Geometry check sheet. Reference: the model listing, model coordinates, mm. Face numbers are marked on the shaded views. A direction names the side the tool comes from. Round coordinates to 2 decimals unless told otherwise and drop trailing zeros. Write each loop counter-clockwise with the first axis right and the second up, starting at its lowest first coordinate (ties: lowest second). Pieces come first, ordered by that corner, then holes. Notation, with made-up numbers: (47.5, 0.25) - (53.5, 0.25) arc R28 ccw to (53.5, 33.25) - close; hole circle Ø9 at (88, 43.25). An arc over 180 degrees is marked (long way). Return JSON: item names as keys, results as strings. Group by question number.
from build123d import *

# Parameters (mm, degrees)
CROQUIS1_R                 = 13
SALIENTE_EXTRUIR1_DEPTH    = 62
CROQUIS2_R                 = 5
CORTAR_EXTRUIR1_DEPTH      = 62
CROQUIS3_R                 = 2.5
CORTAR_EXTRUIR2_DEPTH      = 62
CORTAR_EXTRUIR2_DEPTH_BACK = 62
SALIENTE_EXTRUIR2_DEPTH    = 62
CROQUIS5_W                 = 52
CROQUIS5_H                 = 35
CORTAR_EXTRUIR4_DEPTH      = 62
CROQUIS6_R                 = 2.5
CORTAR_EXTRUIR5_DEPTH      = 62
CROQUIS7_R                 = 5
CORTAR_EXTRUIR6_DEPTH      = 62
CORTAR_EXTRUIR8_DEPTH      = 62
CORTAR_EXTRUIR8_DEPTH_BACK = 62


with BuildPart() as part:
    # Croquis1 → Saliente-Extruir1 (new body)
    with BuildSketch(Plane(origin=(0, 0, 0), x_dir=(0, 0, -1), z_dir=(1, 0, 0))):
        Circle(CROQUIS1_R)
    extrude(amount=SALIENTE_EXTRUIR1_DEPTH)

    # Croquis2 → Cortar-Extruir1 (cut)
    with BuildSketch(Plane(origin=(62, 0, 0), x_dir=(0, 0, -1), z_dir=(1, 0, 0))):
        Circle(CROQUIS2_R)
    extrude(amount=-CORTAR_EXTRUIR1_DEPTH, mode=Mode.SUBTRACT)

    # Croquis3 → Cortar-Extruir2 (cut, two sides)
    with BuildSketch(Plane(origin=(0, 0, 0), x_dir=(1, 0, 0), z_dir=(0, 1, 0))) as cortar_extruir2_sk:
        with Locations((31, 0)):
            Circle(CROQUIS3_R)
    extrude(amount=CORTAR_EXTRUIR2_DEPTH, mode=Mode.SUBTRACT)
    extrude(cortar_extruir2_sk.sketch, amount=-CORTAR_EXTRUIR2_DEPTH_BACK, mode=Mode.SUBTRACT)

    # Croquis4 → Saliente-Extruir2 (add)
    with BuildSketch(Plane(origin=(62, 0, 0), x_dir=(0, 0, -1), z_dir=(1, 0, 0))):
        with BuildLine():
            Line((50, 13), (0, 13))
            ThreePointArc((0, 13), (13, 0), (0, -13))
            Line((0, -13), (50, -13))
            Line((50, -13), (80, -5))
            Line((80, -5), (80, 0))
            Line((80, 0), (80, 5))
            Line((80, 5), (50, 13))
        make_face()
    extrude(amount=-SALIENTE_EXTRUIR2_DEPTH)

    # Croquis5 → Cortar-Extruir4 (cut)
    with BuildSketch(Plane(origin=(0, 13, 0), x_dir=(1, 0, 0), z_dir=(0, 1, 0))):
        with Locations((31, 27.5)):
            Rectangle(CROQUIS5_W, CROQUIS5_H)
    extrude(amount=-CORTAR_EXTRUIR4_DEPTH, mode=Mode.SUBTRACT)

    # Croquis6 → Cortar-Extruir5 (cut)
    with BuildSketch(Plane(origin=(0, 13, 0), x_dir=(1, 0, 0), z_dir=(0, 1, 0))):
        with Locations((31, 0)):
            Circle(CROQUIS6_R)
    extrude(amount=-CORTAR_EXTRUIR5_DEPTH, mode=Mode.SUBTRACT)

    # Croquis7 → Cortar-Extruir6 (cut)
    with BuildSketch(Plane(origin=(0, 0, -80), x_dir=(-1, 0, 0), z_dir=(0, 0, -1))):
        with Locations((-31, 0)):
            Circle(CROQUIS7_R)
    extrude(amount=-CORTAR_EXTRUIR6_DEPTH, mode=Mode.SUBTRACT)

    # Croquis8 → Cortar-Extruir8 (cut, two sides)
    with BuildSketch(Plane(origin=(0, 0, 0), x_dir=(1, 0, 0), z_dir=(0, 1, 0))) as cortar_extruir8_sk:
        Polygon((0, 50), (0, 80), (21, 80), align=None)
        Polygon((41, 80), (62, 50), (62, 80), align=None)
        Polygon((41, 80), (41, 50), (62, 50), align=None)
        Polygon((21, 80), (21, 50), (0, 50), align=None)
    extrude(amount=CORTAR_EXTRUIR8_DEPTH, mode=Mode.SUBTRACT)
    extrude(cortar_extruir8_sk.sketch, amount=-CORTAR_EXTRUIR8_DEPTH_BACK, mode=Mode.SUBTRACT)


solid = part.part
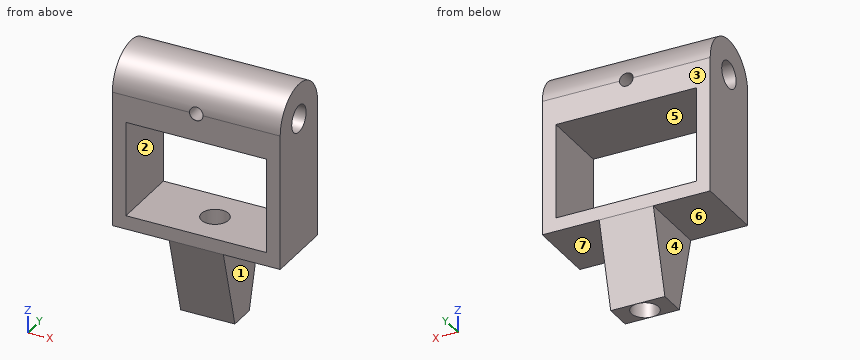
1. Material ranges on line 1 along X through (y, z) = (6.5, 0); line 2 along X through (y, z) = (0, -55.5); line 3 along Y through (x, z) = (47, 0), recorded low to high.
2. Section check B-B (z = -42.5). Enter the section's corners in (x, y).
3. Section check C-C (y = 0). Enter the section's corners in (x, z), and give its area (3 significant figures).
4. Section check A-A (x = 51.5). Enter the section's corners in (y, z), and give its area (3 significant figures).
5. Mould release check, pull along X, two halves, no side actions. Record for the marked faces 1, 2, 3 and 4: pulls with the +X half, pulls with the -X half, needs draft (parallel to the pull), parting line crosses it, or undercut.
6. Tool access check on the marked faces 5, 6 and 7. Record the directions out of +Z, -Z, +X, -X, +Y, -Y that give a thin tool (end or side, any length) a straight path to the whole face; none if there is none.
7. Section check D-D (z = -4). Enter the section's corners in (x, y).
8. Depth check by flat-ended pin: pin 1 Ø3 at (x, z) = (31, 0) entering from +Y; pin 2 Ø3 at (x, z) = (38, 1) entering from -Y; pin 3 Ø13 at (y, z) = (1, -65.5) entering from -X; pin 4 Ø6 at (y, z) = (0, -69) entering from +X. Enter the tip coordinate at first touch or a pass-through.
Result sheet:
{
 "1": {"line 1": "x = 0 to 28.5, 33.5 to 62", "line 2": "x = 21 to 26, 36 to 41", "line 3": "y = -13 to -5, 5 to 13"},
 "2": {"outline": "(0, -13) - (5, -13) - (5, 13) - (0, 13) - close; (57, -13) - (62, -13) - (62, 13) - (57, 13) - close"},
 "3": {"outline": "(0, -50) - (21, -50) - (21, -80) - (26, -80) - (26, -45) - (5, -45) - (5, -10) - (57, -10) - (57, -45) - (36, -45) - (36, -80) - (41, -80) - (41, -50) - (62, -50) - (62, -5) - (0, -5) - close; (0, 5) - (62, 5) - (62, 13) - (0, 13) - close", "area": "1,720 mm²"},
 "4": {"outline": "(-13, -50) - (13, -50) - (13, -45) - (-13, -45) - close; (-13, -10) - (13, -10) - (13, 0) arc R13 ccw to (-13, 0) - close; hole circle Ø10 at (0, 0)", "area": "577 mm²"},
 "5": {"face 1": "pulls with the +X half", "face 2": "undercut", "face 3": "needs draft", "face 4": "pulls with the -X half"},
 "6": {"face 5": "+Y, -Y", "face 6": "-Z, -X, +Y, -Y", "face 7": "-Z, +X, +Y, -Y"},
 "7": {"outline": "(0, -13) - (62, -13) - (62, -3) - (0, -3) - close; (0, 3) - (62, 3) - (62, 13) - (0, 13) - close"},
 "8": {"pin 1": "passes through", "pin 2": "stops at y = -13", "pin 3": "stops at x = 21", "pin 4": "stops at x = 41"}
}
